```python
from build123d import *

# Parameters (mm, degrees)
F0_R     = 3.7
F0_R_2   = 2.2
F1_DEPTH = 5
F2_DEPTH = 3
F3_DEPTH = 3
F5_DEPTH = 2


# Not quite as in the source:
# - a feature of the source that left no trace in its solid (it failed there, or was rolled back) is left out


with BuildPart() as f1:
    # F0 (on Right) → F1 (new body)
    with BuildSketch(Plane.YZ):
        with BuildLine():
            Line((-63.5704365752, 33.3448962937), (-63.5704365752, 5.3711892086))
            Line((-63.5704365752, 5.3711892086), (-33.3704365752, 5.3711892086))
            Line((-33.3704365752, 5.3711892086), (-33.3704365752, 11.9448962937))
            ThreePointArc((-33.3704365752, 11.9448962937), (-35.0704365752, 13.6448962937), (-33.3704365752, 15.3448962937))
            Line((-33.3704365752, 15.3448962937), (-33.3704365752, 20.1448962937))
            ThreePointArc((-33.3704365752, 20.1448962937), (-41.8704365752, 28.6448962937), (-33.3704365752, 37.1448962937))
            Line((-33.3704365752, 37.1448962937), (-33.3704365752, 41.9448962937))
            ThreePointArc((-33.3704365752, 41.9448962937), (-35.0704365752, 43.6448962937), (-33.3704365752, 45.3448962937))
            Line((-33.3704365752, 45.3448962937), (-33.3704365752, 48.3448962937))
            Line((-33.3704365752, 48.3448962937), (-48.5704365752, 48.3448962937))
            Line((-48.5704365752, 48.3448962937), (-63.5704365752, 33.3448962937))
        make_face()
        with Locations((-52.5704365752, 11.0711892086)):
            Circle(F0_R, mode=Mode.SUBTRACT)
        with Locations((-58.5704365752, 23.8448962937)):
            Circle(F0_R_2, mode=Mode.SUBTRACT)
        with BuildLine():
            ThreePointArc((-33.3704365752, 37.1448962937), (-41.8704365752, 28.6448962937), (-33.3704365752, 20.1448962937))
            Line((-33.3704365752, 20.1448962937), (-33.3704365752, 22.6448962937))
            ThreePointArc((-33.3704365752, 22.6448962937), (-39.3704365752, 28.6448962937), (-33.3704365752, 34.6448962937))
            Line((-33.3704365752, 34.6448962937), (-33.3704365752, 37.1448962937))
        make_face()
    extrude(amount=F1_DEPTH)

    # F0 (on Right) → F2 (join)
    with BuildSketch(Plane.YZ):
        with BuildLine():
            Line((-63.5704365752, 33.3448962937), (-63.5704365752, 5.3711892086))
            Line((-63.5704365752, 5.3711892086), (-33.3704365752, 5.3711892086))
            Line((-33.3704365752, 5.3711892086), (-33.3704365752, 11.9448962937))
            ThreePointArc((-33.3704365752, 11.9448962937), (-35.0704365752, 13.6448962937), (-33.3704365752, 15.3448962937))
            Line((-33.3704365752, 15.3448962937), (-33.3704365752, 20.1448962937))
            ThreePointArc((-33.3704365752, 20.1448962937), (-41.8704365752, 28.6448962937), (-33.3704365752, 37.1448962937))
            Line((-33.3704365752, 37.1448962937), (-33.3704365752, 41.9448962937))
            ThreePointArc((-33.3704365752, 41.9448962937), (-35.0704365752, 43.6448962937), (-33.3704365752, 45.3448962937))
            Line((-33.3704365752, 45.3448962937), (-33.3704365752, 48.3448962937))
            Line((-33.3704365752, 48.3448962937), (-48.5704365752, 48.3448962937))
            Line((-48.5704365752, 48.3448962937), (-63.5704365752, 33.3448962937))
        make_face()
        with Locations((-52.5704365752, 11.0711892086)):
            Circle(F0_R, mode=Mode.SUBTRACT)
        with Locations((-58.5704365752, 23.8448962937)):
            Circle(F0_R_2, mode=Mode.SUBTRACT)
        with BuildLine():
            ThreePointArc((-33.3704365752, 15.3448962937), (-35.0704365752, 13.6448962937), (-33.3704365752, 11.9448962937))
            Line((-33.3704365752, 11.9448962937), (-33.3704365752, 15.3448962937))
        make_face()
        with BuildLine():
            ThreePointArc((-33.3704365752, 37.1448962937), (-41.8704365752, 28.6448962937), (-33.3704365752, 20.1448962937))
            Line((-33.3704365752, 20.1448962937), (-33.3704365752, 22.6448962937))
            ThreePointArc((-33.3704365752, 22.6448962937), (-39.3704365752, 28.6448962937), (-33.3704365752, 34.6448962937))
            Line((-33.3704365752, 34.6448962937), (-33.3704365752, 37.1448962937))
        make_face()
        with BuildLine():
            Line((-33.3704365752, 41.9448962937), (-33.3704365752, 45.3448962937))
            ThreePointArc((-33.3704365752, 45.3448962937), (-35.0704365752, 43.6448962937), (-33.3704365752, 41.9448962937))
        make_face()
        with BuildLine():
            ThreePointArc((-33.3704365752, 34.6448962937), (-39.3704365752, 28.6448962937), (-33.3704365752, 22.6448962937))
            Line((-33.3704365752, 22.6448962937), (-33.3704365752, 34.6448962937))
        make_face()
    extrude(amount=F2_DEPTH)

    # F0 (on Right) → F3 (cut, through all)
    with BuildSketch(Plane.YZ):
        with BuildLine():
            ThreePointArc((-33.3704365752, 34.6448962937), (-39.3704365752, 28.6448962937), (-33.3704365752, 22.6448962937))
            Line((-33.3704365752, 22.6448962937), (-33.3704365752, 34.6448962937))
        make_face()
        with BuildLine():
            Line((-33.3704365752, 41.9448962937), (-33.3704365752, 45.3448962937))
            ThreePointArc((-33.3704365752, 45.3448962937), (-35.0704365752, 43.6448962937), (-33.3704365752, 41.9448962937))
        make_face()
        with BuildLine():
            ThreePointArc((-33.3704365752, 15.3448962937), (-35.0704365752, 13.6448962937), (-33.3704365752, 11.9448962937))
            Line((-33.3704365752, 11.9448962937), (-33.3704365752, 15.3448962937))
        make_face()
    extrude(amount=F3_DEPTH, mode=Mode.SUBTRACT)

    # F0 (on Right) → F5 (cut)
    with BuildSketch(Plane.YZ):
        with BuildLine():
            ThreePointArc((-33.3704365752, 37.1448962937), (-41.8704365752, 28.6448962937), (-33.3704365752, 20.1448962937))
            Line((-33.3704365752, 20.1448962937), (-33.3704365752, 22.6448962937))
            ThreePointArc((-33.3704365752, 22.6448962937), (-39.3704365752, 28.6448962937), (-33.3704365752, 34.6448962937))
            Line((-33.3704365752, 34.6448962937), (-33.3704365752, 37.1448962937))
        make_face()
    extrude(amount=F5_DEPTH, mode=Mode.SUBTRACT)


solid = f1.part
```
Source: CAD feature listing. Evaluate the final solid. Frame: model axes, mm. A direction names the side the tool comes from. Give positions to 0.01 mm unless a question says otherwise; leave off trailing zeros. Loops run counter-clockwise (first coordinate to the right, second up) from the corner with the lowest first, then second, coordinate; pieces in that order, holes last. Notation, with made-up numbers: (34.25, 9.5) -> (83.25, 9.5) arc R16 ccw to (83.25, 30.5) -> close; hole circle Ø10 at (-2.75, -6.75). An arc over 180 degrees is marked (long way). Use a Markdown table: item, result. Add a question column.
(1) First-contact query: pin 1 Ø4 at (y, z) = (-36, 25.5) entering from -X; pin 2 Ø1 at (x, z) = (0.5, 35.5) entering from -Y. Flat tips, straight axial feed; report the tip coordinate or a pass-through.
(2) Section query B-B (y = -55). Output: boundary loops of the cut face in (x, z), then the cut area to 3 significant figures.
(3) Access query for faces 4 (the face through (2, -33.37, 47)), 5 (the face through (0.99, -41.87, 28.83)). Directions: +Z, -Z, +X, -X, +Y, -Y. A direction counts if a zero-diameter tool reaches every point of the face in a straight line with its end or side. Return the directions, or none.
(4) Section query A-A (z = 13). Output: boundary loops of the cut face in (x, y), then the cut area to 3 significant figures.
(5) Pull-direction query (Z, two-part tool) for faces 1 (the face through (2, -40, 29)), 2 (the face through (2, -63.57, 20)), 3 (the face through (2.465, -55.965, 40.95)); classes: +Z half, -Z half, draft (parallel to the pull), parting line (faces both ways), or undercut.
(6) Ray query, line 1 (Y direction, x = 0.3, z = 29); line 2 (Z direction, x = 0.3, y = -38.5); line 3 (Y direction, x = 4.6, z = 11). Return the intervals inside material, ascending.
(7) Section query D-D (x = 3.9). Output: boundary loops of the cut face in (y, z), then the cut area to 3 significant figures.
(8) Section query C-C (x = 0.6). Output: boundary loops of the cut face in (y, z), then the cut area to 3 significant figures.
Checked values:
| question | item | result |
|---|---|---|
| 1 | pin 1 | x = 2 |
| 1 | pin 2 | y = -61.92 |
| 2 | outline | (0, 5.37) -> (5, 5.37) -> (5, 8.28) -> (0, 8.28) -> close; (0, 13.86) -> (5, 13.86) -> (5, 41.92) -> (0, 41.92) -> close |
| 2 | area | 155 mm^2 |
| 3 | face 4 | +Z, -Z, +X, -X, +Y |
| 3 | face 5 | -X, +Y |
| 4 | outline | (0, -63.57) -> (5, -63.57) -> (5, -55.73) -> (0, -55.73) -> close; (0, -49.41) -> (5, -49.41) -> (5, -34.94) -> (0, -34.94) -> close |
| 4 | area | 112 mm^2 |
| 5 | face 1 | undercut |
| 5 | face 2 | draft |
| 5 | face 3 | +Z half |
| 6 | line 1 | -63.57 to -41.86 |
| 6 | line 2 | 5.37 to 21.87, 35.42 to 48.34 |
| 6 | line 3 | -63.57 to -56.27, -48.87 to -33.37 |
| 7 | outline | (-63.57, 5.37) -> (-33.37, 5.37) -> (-33.37, 11.94) arc R1.7 cw to (-33.37, 15.34) -> (-33.37, 22.64) arc R6 cw to (-33.37, 34.64) -> (-33.37, 41.94) arc R1.7 cw to (-33.37, 45.34) -> (-33.37, 48.34) -> (-48.57, 48.34) -> (-63.57, 33.34) -> close; hole circle Ø4.4 at (-58.57, 23.84); hole circle Ø7.4 at (-52.57, 11.07) |
| 7 | area | 1,060 mm^2 |
| 8 | outline | (-63.57, 5.37) -> (-33.37, 5.37) -> (-33.37, 11.94) arc R1.7 cw to (-33.37, 15.34) -> (-33.37, 20.14) arc R8.5 cw to (-33.37, 37.14) -> (-33.37, 41.94) arc R1.7 cw to (-33.37, 45.34) -> (-33.37, 48.34) -> (-48.57, 48.34) -> (-63.57, 33.34) -> close; hole circle Ø4.4 at (-58.57, 23.84); hole circle Ø7.4 at (-52.57, 11.07) |
| 8 | area | 1,000 mm^2 |
